Source: three-view drawing plus pictorial views. Frame: mm from the lowest corner of the part. Round coordinates to 2 decimals unless told otherwise and drop trailing zeros. Loops run counter-clockwise (first coordinate to the right, second up) from the corner with the lowest first, then second, coordinate; pieces in that order, holes last. Notation, with made-up numbers: M -15,63.5 L 0,63.5 A12 ccw 0,79.5 Z; hole C 61.25,88 d7. An arc over 180 degrees is marked long. Return JSON: item names as keys, results as strings. Group by question number.
1) Section C-C (x = 80.5). Output: boundary loops of the cut face in (y, z).
2) Section A-A (y = 32). Output: boundary loops of the cut face in (x, z).
3) Material intervals for line 1 (Z direction, x = 93, y = 155.5); line 2 (X direction, y = 162.5, z = 177); line 3 (X direction, y = 19, z = 314), sorted ascending. Write a range as from..to.
4) Section B-B (z = 164). Output: boundary loops of the cut face in (x, y).
5) Contact query for flat-ended pins moving along their axis: P1, Ø4, axis at x = 424.5, y = 167, coming from the +Z side; P2, Ø10, axis at y = 167, z = 323, coming from the +X side; P3, Ø7.5, axis at x = 418, z = 109, coming from the -Y side. Output: stop coordinate, or through.
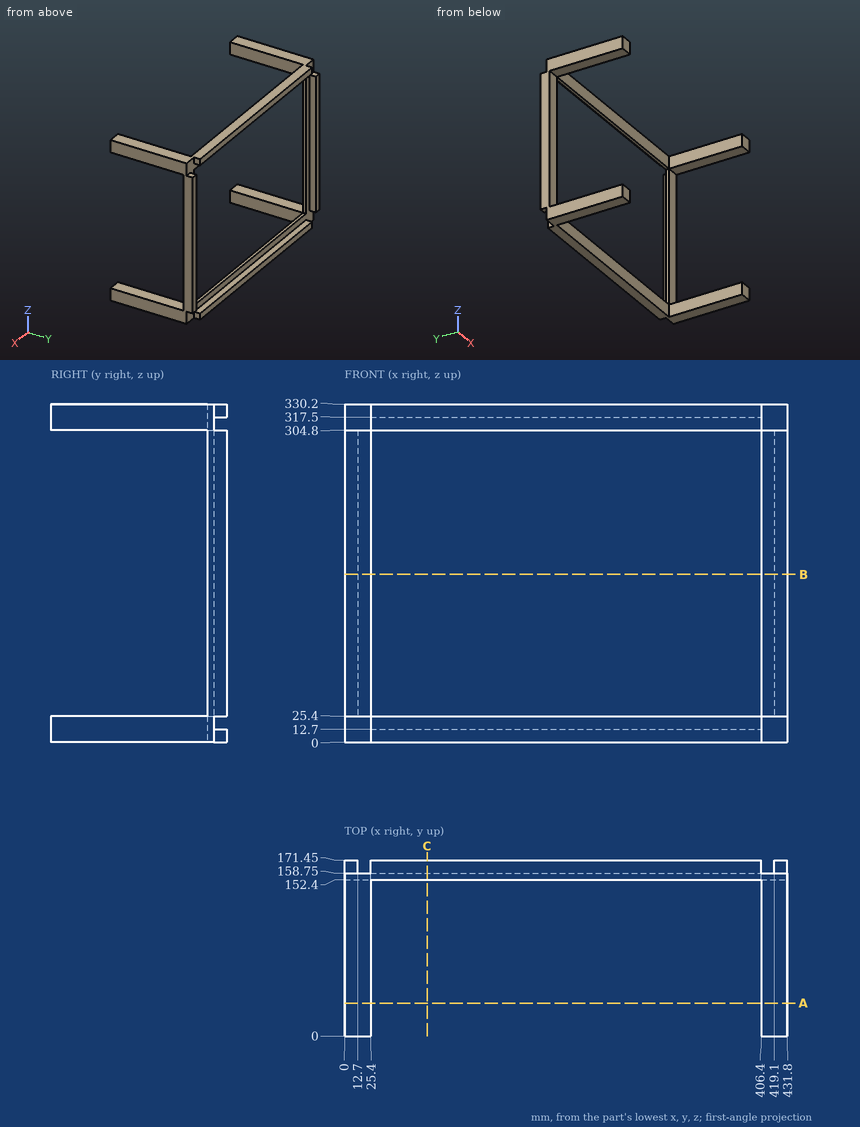
Returned:
{
 "1": {"outline": "M 152.4,0 L 171.45,0 L 171.45,12.7 L 158.75,12.7 L 158.75,25.4 L 152.4,25.4 Z; M 152.4,304.8 L 158.75,304.8 L 158.75,317.5 L 171.45,317.5 L 171.45,330.2 L 152.4,330.2 Z"},
 "2": {"outline": "M 0,0 L 25.4,0 L 25.4,25.4 L 0,25.4 Z; M 0,304.8 L 25.4,304.8 L 25.4,330.2 L 0,330.2 Z; M 406.4,0 L 431.8,0 L 431.8,25.4 L 406.4,25.4 Z; M 406.4,304.8 L 431.8,304.8 L 431.8,330.2 L 406.4,330.2 Z"},
 "3": {"line 1": "z = 0..25.4, 304.8..330.2", "line 2": "x = 0..12.7, 419.1..431.8", "line 3": "x = 0..25.4, 406.4..431.8"},
 "4": {"outline": "M 0,152.4 L 25.4,152.4 L 25.4,158.75 L 12.7,158.75 L 12.7,171.45 L 0,171.45 Z; M 406.4,152.4 L 431.8,152.4 L 431.8,171.45 L 419.1,171.45 L 419.1,158.75 L 406.4,158.75 Z"},
 "5": {"P1": "stops at z = 304.8", "P2": "stops at x = 406.4", "P3": "stops at y = 152.4"}
}
